Geometry: see drawing. Coordinates: mm, zero at the bounding-box minimum. A direction names the side the tool comes from. Give positions to 0.01 mm unless a question says otherwise; leave off trailing zeros. Order: outer loops, then holes, each group sorted by start corner. A loop starts at its lowest first (then second) coordinate and runs counter-clockwise, first axis right, second up. Notation, with made-up numbers: (-39, 46) - (-8, 46) arc R24 ccw to (-8, 85) - close; hole circle Ø5 at (-5, -33.5). An arc over 180 degrees is marked (long way). Write item = value, one per line. Start each with the question number.
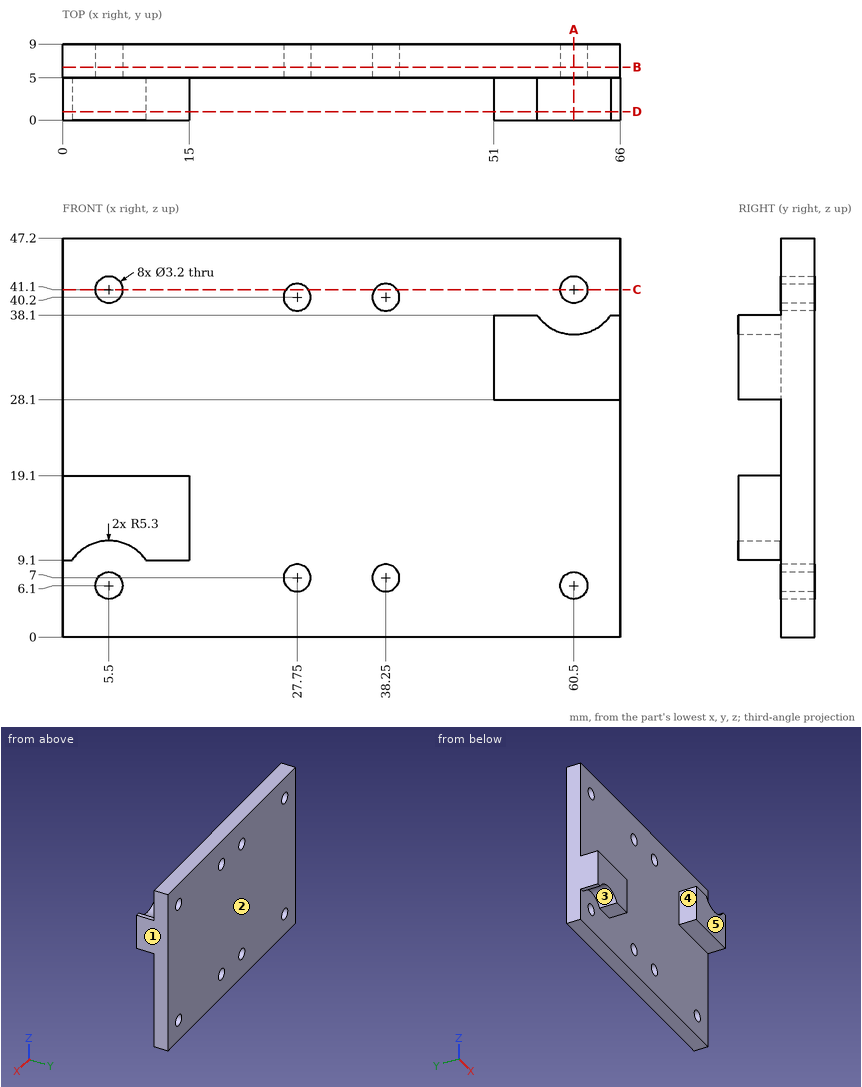
Q1. Contact query for flat-ended pins moving along their axis: pin 1 (3 mm diameter, centred on x = 38.25, z = 40.2, fed in from +Y) (3 decimals); pin 2 (8 mm diameter, centred on x = 18.5, z = 31, fed in from -Y); pin 3 (2 mm diameter, centred on y = 3, z = 16, fed in from +X); pin 4 (2.5 mm diameter, centred on y = 2, z = 33, fed in from -X). Output: stop coordinate, or through.
Q2. Material intervals for line 1 along X through (y, z) = (7.4, 6.1); line 2 along X through (y, z) = (8.1, 40.2); line 3 along Z through (x, y) = (38, 7.5), sorted ascending. Write a range as from..to.
Q3. Pull-direction query (X, two-part tool) for the marked faces 1, 2 and 3; classes: +X half, -X half, draft (parallel to the pull), parting line (faces both ways), or undercut.
Q4. Section C-C, the plane z = 41.1. Return the cut outline in (x, y), then the cut area to 3 significant figures.
Q5. Section A-A, the plane x = 60.5. Return the cut outline in (y, z).
Q6. Section D-D, the plane y = 1. Return the cut outline in (x, z).
Q7. Section B-B, the plane y = 6.25. Count the separate pieces of the cut face and the enclosed holes in it, then the cut area to 3 significant figures.
Q8. Set-up query: the marked faces 4 and 5. Return all of +Z, -Z, +X, -X, +Y, -Y with unobstructed straight access to the full face (end or side cutting, diameter ignored); none if empty.
The answers:
q1.pin_1 = through
q1.pin_2 = 5
q1.pin_3 = 15
q1.pin_4 = 51
q2.line_1 = 0..3.9, 7.1..26.43, 29.07..36.93, 39.57..58.9, 62.1..66
q2.line_2 = 0..4.18, 6.82..26.15, 29.35..36.65, 39.85..59.18, 61.82..66
q2.line_3 = 0..5.42, 8.58..38.62, 41.78..47.2
q3.face_1 = +X half
q3.face_2 = draft
q3.face_3 = undercut
q4.outline = (0, 5) - (3.9, 5) - (3.9, 9) - (0, 9) - close; (7.1, 5) - (26.43, 5) - (26.43, 9) - (7.1, 9) - close; (29.07, 5) - (36.93, 5) - (36.93, 9) - (29.07, 9) - close; (39.57, 5) - (58.9, 5) - (58.9, 9) - (39.57, 9) - close; (62.1, 5) - (66, 5) - (66, 9) - (62.1, 9) - close
q4.area = 217 mm²
q5.outline = (0, 28.1) - (5, 28.1) - (5, 7.7) - (9, 7.7) - (9, 39.5) - (5, 39.5) - (5, 35.8) - (0, 35.8) - close; (5, 0) - (9, 0) - (9, 4.5) - (5, 4.5) - close; (5, 42.7) - (9, 42.7) - (9, 47.2) - (5, 47.2) - close
q6.outline = (0, 9.1) - (1.13, 9.1) arc R5.3 cw to (9.87, 9.1) - (15, 9.1) - (15, 19.1) - (0, 19.1) - close; (51, 28.1) - (66, 28.1) - (66, 38.1) - (64.87, 38.1) arc R5.3 cw to (56.13, 38.1) - (51, 38.1) - close
q7.separate_pieces = 1
q7.enclosed_holes = 8
q7.area = 3,050 mm²
q8.face_4 = +Z, -Z, -X, -Y
q8.face_5 = +Z, -Z, +X, -X, -Y
